Print and shaded views of the part. All mm, measured from the part's lowest x, y and z. Round coordinates to 2 decimals unless told otherwise and drop trailing zeros. Write each loop counter-clockwise with the first axis right and the second up, starting at its lowest first coordinate (ties: lowest second). Pieces come first, ordered by that corner, then holes. Notation, with made-up numbers: M 15.25,10 L 55.25,10 A29 ccw 55.25,40 Z; hole C 41.5,85.5 d10. An arc over 180 degrees is marked long. Write item = value, one per line.
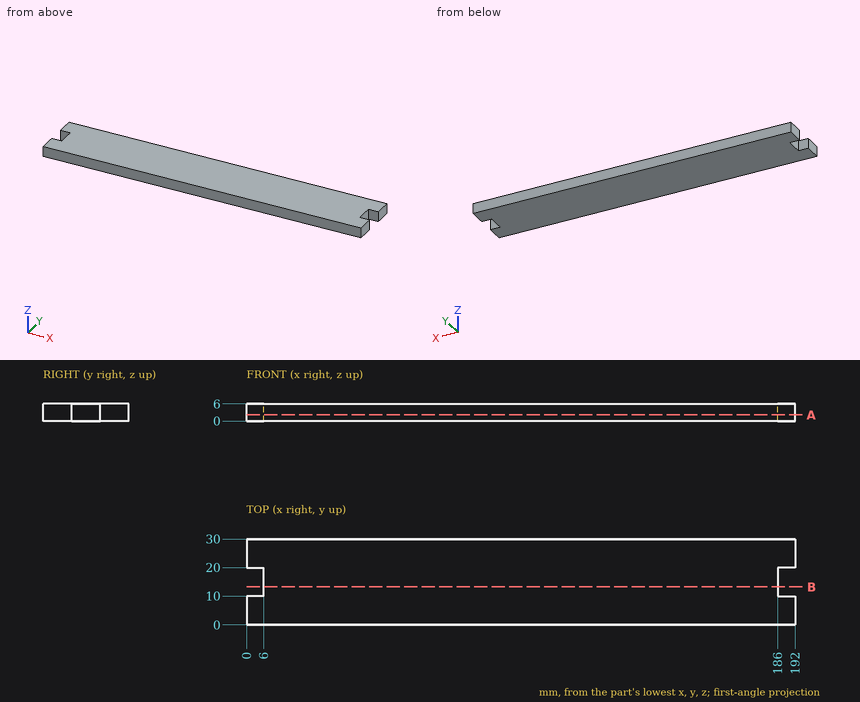
1. Flat gauge pins, fed straight in: pin 1 (3 mm diameter, centred on y = 13.5, z = 3.5, fed in from +X); pin 2 (3 mm diameter, centred on y = 15.5, z = 3.5, fed in from -X). Where does each tip first touch, or does it go through?
Responses:
pin_1 = 186
pin_2 = 6
2. Band-saw the part on A-A (z = 2.2). List the corners of the cut face in (x, y).
Responses:
outline = M 0,0 L 192,0 L 192,10 L 186,10 L 186,20 L 192,20 L 192,30 L 0,30 L 0,20 L 6,20 L 6,10 L 0,10 Z
3. Probe probe 1 along X at (y, z) = (19.75, 3.05). List the from-to ranges inside material, lowest first.
Responses:
probe_1 = 6 to 186
4. Band-saw the part on B-B (y = 13.25). List the corners of the cut face in (x, z), plus the area to 3 significant figures.
Responses:
outline = M 6,0 L 186,0 L 186,6 L 6,6 Z
area = 1,080 mm²
